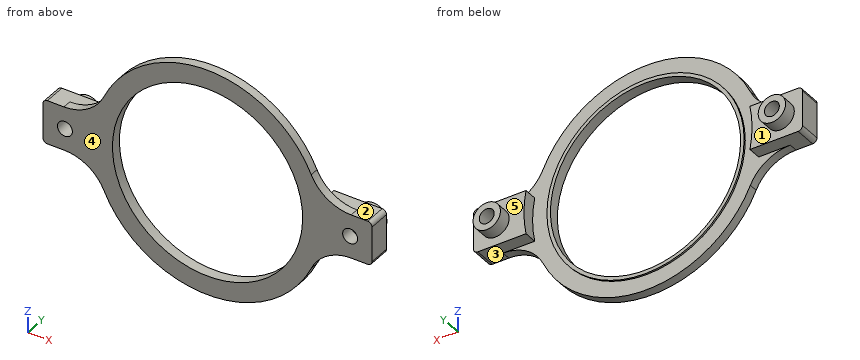
```python
from build123d import *

# Parameters (mm, degrees)
SKETCH1_R            = 26
SKETCH1_R_2          = 21.675
BOSS_EXTRUDE1_DEPTH  = 2
SKETCH2_R            = 22.475
SKETCH2_R_2          = 21.675
BOSS_EXTRUDE2_DEPTH  = 0.4
BOSS_EXTRUDE3_DEPTH  = 5
SKETCH4_W            = 10
SKETCH4_H            = 2
BOSS_EXTRUDE4_DEPTH  = 9.9853
SKETCH5_R            = 3.125
BOSS_EXTRUDE7_DEPTH  = 5
M3_CLEARANCE_HOLE1_D = 3.4
FILLET1_R            = 1
SKETCH9_R            = 1.7
BOSS_EXTRUDE8_DEPTH  = 3
FILLET3_R            = 10


with BuildPart() as part:
    # Sketch1 → Boss-Extrude1 (new body)
    with BuildSketch(Plane(origin=(0, 0, 0), x_dir=(1, 0, 0), z_dir=(0, 1, 0))):
        with Locations(Location((0, 0, 0), (0, 0, 270))):
            Circle(SKETCH1_R)
        with Locations(Location((0, 0, 0), (0, 0, 270))):
            Circle(SKETCH1_R_2, mode=Mode.SUBTRACT)
    extrude(amount=BOSS_EXTRUDE1_DEPTH)

    # Sketch2 → Boss-Extrude2 (add)
    with BuildSketch(Plane(origin=(0, 2, 0), x_dir=(1, 0, 0), z_dir=(0, 1, 0))):
        with Locations(Location((0, 0, 0), (0, 0, 270))):
            Circle(SKETCH2_R)
        with Locations(Location((0, 0, 0), (0, 0, 270))):
            Circle(SKETCH2_R_2, mode=Mode.SUBTRACT)
    extrude(amount=BOSS_EXTRUDE2_DEPTH)

    # Sketch3 → Boss-Extrude3 (add)
    with BuildSketch(Plane.XZ):
        with BuildLine():
            Line((25.514701644, -5), (27.514701644, -5))
            Line((27.514701644, -5), (27.514701644, 5))
            Line((27.514701644, 5), (25.514701644, 5))
            ThreePointArc((25.514701644, 5), (26, 0), (25.514701644, -5))
        make_face()
    boss_extrude3 = extrude(amount=-BOSS_EXTRUDE3_DEPTH)

    # Sketch4 → Boss-Extrude4 (add)
    with BuildSketch(Plane(origin=(27.514701644, 0, 0), x_dir=(0, 0, -1), z_dir=(1, 0, 0))):
        with Locations((0, 4)):
            Rectangle(SKETCH4_W, SKETCH4_H)
    boss_extrude4 = extrude(amount=BOSS_EXTRUDE4_DEPTH)

    # Sketch5 → Boss-Extrude7 (add)
    with BuildSketch(Plane.XZ.offset(-3)):
        with Locations(Location((32.500001644, 0, 0), (0, 0, 270))):
            Circle(SKETCH5_R)
    boss_extrude7 = extrude(amount=-BOSS_EXTRUDE7_DEPTH)

    # M3 Clearance Hole1 (through all)
    with Locations(Plane.XZ.offset(-3)):
        with Locations((32.500001644, 0)):
            m3_clearance_hole1 = Hole(M3_CLEARANCE_HOLE1_D / 2)

    # Mirror1: Boss-Extrude3, Boss-Extrude4, Boss-Extrude7, M3 Clearance Hole1 across plane
    add(boss_extrude3.mirror(Plane(origin=(0, 0, 0), x_dir=(0, 0, 1), z_dir=(1, 0, 0))))
    add(boss_extrude4.mirror(Plane(origin=(0, 0, 0), x_dir=(0, 0, 1), z_dir=(1, 0, 0))))
    add(boss_extrude7.mirror(Plane(origin=(0, 0, 0), x_dir=(0, 0, 1), z_dir=(1, 0, 0))))
    add(m3_clearance_hole1.mirror(Plane(origin=(0, 0, 0), x_dir=(0, 0, 1), z_dir=(1, 0, 0))), mode=Mode.SUBTRACT)

    # Fillet1
    fillet1_edges = [part.edges().sort_by_distance(p)[0] for p in [
        (37.500001644, 4, -5),
        (37.500001644, 4, 5),
        (-37.500001644, 4, -5),
        (-37.500001644, 4, 5),
    ]]
    fillet(fillet1_edges, radius=FILLET1_R)

    # Sketch9 → Boss-Extrude8 (add, through all)
    with BuildSketch(Plane.XZ.offset(-3)):
        with BuildLine():
            Line((-37.500001644, 4), (-37.500001644, -4))
            ThreePointArc((-37.500001644, -4), (-37.207108426, -4.707106781), (-36.500001644, -5))
            Line((-36.500001644, -5), (-27.514701644, -5))
            Line((-27.514701644, -5), (-27.514701644, 5))
            Line((-27.514701644, 5), (-36.500001644, 5))
            ThreePointArc((-36.500001644, 5), (-37.207108426, 4.707106781), (-37.500001644, 4))
        make_face()
        with Locations(Location((-32.500001644, 0, 0), (0, 0, 270))):
            Circle(SKETCH9_R, mode=Mode.SUBTRACT)
        with BuildLine():
            Line((37.500001644, -4), (37.500001644, 4))
            ThreePointArc((37.500001644, 4), (37.207108426, 4.707106781), (36.500001644, 5))
            Line((36.500001644, 5), (27.514701644, 5))
            Line((27.514701644, 5), (27.514701644, -5))
            Line((27.514701644, -5), (36.500001644, -5))
            ThreePointArc((36.500001644, -5), (37.207108426, -4.707106781), (37.500001644, -4))
        make_face()
        with Locations(Location((32.500001644, 0, 0), (0, 0, 270))):
            Circle(SKETCH9_R, mode=Mode.SUBTRACT)
    extrude(amount=BOSS_EXTRUDE8_DEPTH)

    # Fillet3
    fillet3_edges = [part.edges().sort_by_distance(p)[0] for p in [
        (25.514701644, 1, -5),
        (25.514701644, 1, 5),
        (-25.514701644, 1, 5),
        (-25.514701644, 1, -5),
    ]]
    fillet(fillet3_edges, radius=FILLET3_R)


solid = part.part
```
Geometry: final body of the model. Coordinates: model frame, mm. Face numbers are marked on the shaded views. A direction names the side the tool comes from. Give positions to 0.01 mm unless a question says otherwise; leave off trailing zeros. Order: outer loops, then holes, each group sorted by start corner. A loop starts at its lowest first (then second) coordinate and runs counter-clockwise, first axis right, second up. Notation, with made-up numbers: (24, 42.25) -> (45, 42.25) arc R17 cw to (45, 66.25) -> close; hole circle Ø2 at (77.25, -36.75). An arc over 180 degrees is marked (long way). Write each question's results on one line, items separated by ' | '. Start each with the question number.
1) Section D-D (z = 6). Return loops of the section in (x, y), then the cut area to 3 significant figures.
2) Set-up query: the marked faces 3, 4 and 5. Return all of +Z, -Z, +X, -X, +Y, -Y with unobstructed straight access to the full face (end or side cutting, diameter ignored); none if empty.
3) Section A-A (y = 1). Return loops of the section in (x, z) (3 decimals), then the cut area to 3 significant figures.
4) Section B-B (x = 0). Return loops of the section in (y, z) (3 decimals), then the cut area to 3 significant figures.
5) Line query: line 1 (X direction, y = 4.2, z = 0); line 2 (X direction, y = 1.8, z = 0) (3 decimals); line 3 (X direction, y = 2.3, z = 0) (3 decimals). Output: solid intervals per line, ascending. Write a range as from..to.
6) First-contact query: pin 1 (4 mm diameter, centred on y = 2.5, z = -5, fed in from +X); pin 2 (1.5 mm diameter, centred on x = 33.5, y = 3, fed in from +Z); pin 3 (1.5 mm diameter, centred on x = -29.5, y = 2, fed in from +Z); pin 4 (4 mm diameter, centred on x = -28.5, y = 3.5, fed in from -Z). Flat tips, straight axial feed; report the tip coordinate or a pass-through.
7) Section C-C (z = 0). Count the separate pieces of the cut face and the enclosed holes in it, then the cut area to 3 significant figures.
8) Draft query along X for the marked faces 1 and 2. Return one class per face: pulls with the +X half, pulls with the -X half, needs draft (parallel to the pull), parting line crosses it, or undercut.
Calculated:
1) outline: (-28.37, 0) -> (-20.83, 0) -> (-20.83, 2.4) -> (-21.66, 2.4) -> (-21.66, 2) -> (-28.37, 2) -> close; (20.83, 0) -> (28.37, 0) -> (28.37, 2) -> (21.66, 2) -> (21.66, 2.4) -> (20.83, 2.4) -> close | area: 30.8 mm2
2) face 3: -Z, +X, +Y | face 4: +Z, -Z, +X, -X, -Y | face 5: +Y
3) outline: (-37.5, -4) arc R1 ccw to (-36.5, -5) -> (-32.726, -5) arc R10 cw to (-23.636, -10.833) arc R26 ccw to (23.636, -10.833) arc R10 cw to (32.726, -5) -> (36.5, -5) arc R1 ccw to (37.5, -4) -> (37.5, 4) arc R1 ccw to (36.5, 5) -> (32.726, 5) arc R10 cw to (23.636, 10.833) arc R26 ccw to (-23.636, 10.833) arc R10 cw to (-32.726, 5) -> (-36.5, 5) arc R1 ccw to (-37.5, 4) -> close; hole circle Ø3.4 at (-32.5, 0); hole circle Ø43.35 at (0, 0); hole circle Ø3.4 at (32.5, 0) | area: 897 mm2
4) outline: (0, -26) -> (2, -26) -> (2, -22.475) -> (2.4, -22.475) -> (2.4, -21.675) -> (0, -21.675) -> close; (0, 21.675) -> (2.4, 21.675) -> (2.4, 22.475) -> (2, 22.475) -> (2, 26) -> (0, 26) -> close | area: 17.9 mm2
5) line 1: -37.5..-34.2, -30.8..-26, 26..30.8, 34.2..37.5 | line 2: -37.5..-34.2, -30.8..-21.675, 21.675..30.8, 34.2..37.5 | line 3: -37.5..-34.2, -30.8..-26, -22.475..-21.675, 21.675..22.475, 26..30.8, 34.2..37.5
6) pin 1: x = 37.5 | pin 2: z = 5 | pin 3: z = 5.82 | pin 4: z = -6.68
7) separate pieces: 4 | enclosed holes: 0 | area: 116 mm2
8) face 1: undercut | face 2: needs draft
